from build123d import *

# Parameters (mm, degrees)
BOSS_EXTRUDE1_DEPTH = 5.5
CUT_EXTRUDE1_REACH  = 10.602
SKETCH2_R           = 3


with BuildPart() as part:
    # Sketch1 → Boss-Extrude1 (new body)
    with BuildSketch(Plane(origin=(0, 0, 0), x_dir=(0, 1, 0), z_dir=(0, 0, 1))):
        Polygon((5, 0), (2.5, 4.330127019), (-2.5, 4.330127019), (-5, 0), (-2.5, -4.330127019), (2.5, -4.330127019), align=None)
    extrude(amount=BOSS_EXTRUDE1_DEPTH)

    # Sketch2 → Cut-Extrude1 (cut, up to next)
    with BuildSketch(Plane.XY.offset(5.5), mode=Mode.PRIVATE) as cut_extrude1_sk1:
        Circle(SKETCH2_R)
    cut_extrude1_tool1 = extrude(cut_extrude1_sk1.sketch, amount=-CUT_EXTRUDE1_REACH, mode=Mode.PRIVATE) & part.part
    add(cut_extrude1_tool1.solids().sort_by_distance((0, 0, 5.5))[0], mode=Mode.SUBTRACT)


solid = part.part
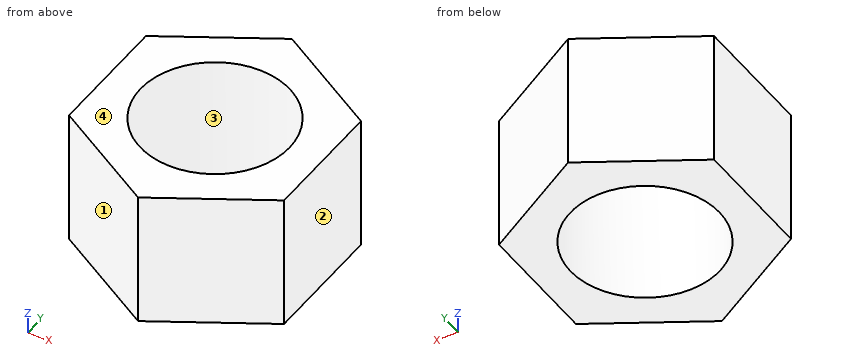
Here's how the part is built. I have some questions about the finished solid (model axes, mm). Face numbers are marked on the shaded views. Coordinates: 2 decimals unless noted, no trailing zeros. Order: outer loops, then holes, each group sorted by start corner. A loop starts at its lowest first (then second) coordinate and runs counter-clockwise, first axis right, second up. Notation, with made-up numbers: (55, 84.5) - (94, 84.5) arc R33 ccw to (94, 114.5) - close; hole circle Ø3 at (3.5, 4). An arc over 180 degrees is marked (long way). Use CSV: the item, a comma, the result in double quotes. Start each with the question number.
1. If we mould it in two halves opening along X, with no side actions, what happens to the marked faces 1, 2, 3 and 4? For each: +X half, -X half, draft (parallel to the pull), parting line (faces both ways), or undercut.
2. Suppose I cut it at C-C on x = 2. List the corners of the cut face in (y, z) for me, then the cut area to 3 significant figures.
3. Suppose I cut it at D-D on y = -3.5. List the corners of the cut face in (x, z) for me, then the cut area to 3 significant figures.
4. Please list where these lines run through material, in increasing order: line 1 (X direction, y = 2, z = 5.15); line 2 (X direction, y = 0.5, z = 2.2); line 3 (Y direction, x = -1.75, z = 3.35). Write a range as from..to.
5. Suppose I cut it at B-B on y = 1.75. List the corners of the cut face in (x, z) for me, then the cut area to 3 significant figures.
6. Suppose I cut it at A-A on z = 3.75. List the corners of the cut face in (x, y) for me, then the cut area to 3 significant figures.
7. I'm going to push flat-ended pins straight in: pin 1 (2 mm diameter, centred on x = -3, z = 4.5, fed in from +Y); pin 2 (1.5 mm diameter, centred on x = -3, z = 3.5, fed in from +Y); pin 3 (3.5 mm diameter, centred on x = 0, y = 0, fed in from +Z); pin 4 (2 mm diameter, centred on x = -2.5, z = 1, fed in from -Y). Where does each tip first touch, or does it pass through?
Output:
1,face 1,"-X half"
1,face 2,"+X half"
1,face 3,"undercut"
1,face 4,"draft"
2,outline,"(-3.85, 0) - (-2.24, 0) - (-2.24, 5.5) - (-3.85, 5.5) - close; (2.24, 0) - (3.85, 0) - (3.85, 5.5) - (2.24, 5.5) - close"
2,area,"17.7 mm2"
3,outline,"(-2.6, 0) - (2.6, 0) - (2.6, 5.5) - (-2.6, 5.5) - close"
3,area,"28.6 mm2"
4,line 1,"x = -4.33..-2.24, 2.24..4.33"
4,line 2,"x = -4.33..-2.96, 2.96..4.33"
4,line 3,"y = -3.99..-2.44, 2.44..3.99"
5,outline,"(-4.33, 0) - (-2.44, 0) - (-2.44, 5.5) - (-4.33, 5.5) - close; (2.44, 0) - (4.33, 0) - (4.33, 5.5) - (2.44, 5.5) - close"
5,area,"20.8 mm2"
6,outline,"(-4.33, -2.5) - (0, -5) - (4.33, -2.5) - (4.33, 2.5) - (0, 5) - (-4.33, 2.5) - close; hole circle Ø6 at (0, 0)"
6,area,"36.7 mm2"
7,pin 1,"stops at y = 3.85"
7,pin 2,"stops at y = 3.7"
7,pin 3,"passes through"
7,pin 4,"stops at y = -4.13"
